Work out the finished part from the listing and answer in its coordinate system (mm). A direction names the side the tool comes from. Coordinates: 2 decimals unless noted, no trailing zeros. Loops run counter-clockwise (first coordinate to the right, second up) from the corner with the lowest first, then second, coordinate; pieces in that order, holes last.
```python
from build123d import *

# Parameters (mm, degrees)
F1_DEPTH       = 7.5
F2_DEPTH       = 2.5
F4_D           = 5.5
F4_DEPTH       = 8
F4_CSINK_D     = 11.2
F4_CSINK_ANGLE = 90
F4_TIP         = 1.6523667023


with BuildPart() as f1:
    # F0 (on Top) → F1 (new body, symmetric)
    with BuildSketch(Plane.XY):
        Polygon((2, 28.0777472107), (2, 40), (-2, 40), (-2, -40), (2, -40), (2, -28.0777472107), (2, -3.9222527893), (2, 3.9222527893), align=None)
    extrude(amount=F1_DEPTH, both=True)

    # F0 (on Top) → F2 (join, symmetric)
    with BuildSketch(Plane.XY):
        with BuildLine():
            Line((21, 28.0777472107), (2, 28.0777472107))
            Line((2, 28.0777472107), (2, 3.9222527893))
            Line((2, 3.9222527893), (21, 3.9222527893))
            Line((21, 3.9222527893), (21, 7.9222527893))
            ThreePointArc((21, 7.9222527893), (6.5, 16), (21, 24.0777472107))
            Line((21, 24.0777472107), (21, 28.0777472107))
        make_face()
        with BuildLine():
            Line((21, -3.9222527893), (2, -3.9222527893))
            Line((2, -3.9222527893), (2, -28.0777472107))
            Line((2, -28.0777472107), (21, -28.0777472107))
            Line((21, -28.0777472107), (21, -24.0777472107))
            ThreePointArc((21, -24.0777472107), (6.5, -16), (21, -7.9222527893))
            Line((21, -7.9222527893), (21, -3.9222527893))
        make_face()
    extrude(amount=F2_DEPTH, both=True)

    # F4
    with Locations(Plane.YZ.offset(2)):
        with Locations((-34.0387472107, 0), (34.0387472107, 0)):
            CounterSinkHole(F4_D / 2, F4_CSINK_D / 2, depth=F4_DEPTH, counter_sink_angle=F4_CSINK_ANGLE)
            with Locations((0, 0, -(F4_DEPTH + F4_TIP / 2))):  # 118° drill point
                Cone(0, F4_D / 2, F4_TIP, mode=Mode.SUBTRACT)


solid = f1.part
```
1. A cutting plane is placed at C-C, the plane y = -16. Give the vertices of the cut face in (x, z).
2. Straight lines are drawn through the part: probe 1 along Y at (x, z) = (-1.3, 0); probe 2 along Y at (x, z) = (16, -1.15); probe 3 along X at (y, z) = (28.5, -6). For each, find the intervals that lie inside material, in ascending order.
3. For faces 5 (the conical face through (-0.712, -36.794, 0.868)), 6 (the flat face through (5, -16, 2.5)), 7 (the flat face through (12, -3.922, 0)), 8 (the flat face through (5, 16, -2.5)), 9 (the cylindrical face through (6.504, -16.283, 0.035)), determine the directions among +Z, -Z, +X, -X, +Y, -Y from which every point of the face is accessible in a straight line to the end or side of a thin tool.
4. Each of these flat-tipped pins is pushed along its axis until it touches: P1, Ø9.5, axis at x = 9.5, y = 15, coming from the -Z side; P2, Ø6, axis at x = 10, z = 1, coming from the +Y side; P3, Ø1.5, axis at x = 8, z = -0.5, coming from the -Y side. Where does it stop, or does it pass through?
5. Determine the mould class of faces 1 (the flat face through (0, -40, 0)), 2 (the cylindrical face through (6.504, 15.717, -0.035)), 3 (the flat face through (11, 3.922, 0)), 4 (the flat face through (21, 26, 0)) for opening direction Y: released by +Y, released by -Y, zero draft, split by the parting line, or undercut.
6. A cutting plane is placed at D-D, the plane x = 0.25. Give the vertices of the cut face in (y, z), then the cut area to 3 significant figures.
7. A cutting plane is placed at A-A, the plane x = 16. Give the vertices of the cut face in (y, z), then the cut area to 3 significant figures.
8. A cutting plane is placed at B-B, the plane z = 0. Give the vertices of the cut face in (x, y), then the cut area to 3 significant figures.
Answers below:
1. outline: (-2, -7.5) - (2, -7.5) - (2, -2.5) - (6.5, -2.5) - (6.5, 2.5) - (2, 2.5) - (2, 7.5) - (-2, 7.5) - close
2. probe 1: y = -40 to -36.79, -31.29 to 31.29, 36.79 to 40
2. probe 2: y = -28.08 to -25.5, -6.5 to -3.92, 3.92 to 6.5, 25.5 to 28.08
2. probe 3: x = -2 to 2
3. face 5: +X
3. face 6: +Z, +X, +Y, -Y
3. face 7: +Z, -Z, +X
3. face 8: -Z, +X, +Y, -Y
3. face 9: +Z, -Z
4. P1: stops at z = -2.5
4. P2: stops at y = 28.08
4. P3: stops at y = -28.08
5. face 1: released by -Y
5. face 2: undercut
5. face 3: undercut
5. face 4: zero draft
6. outline: (-40, -7.5) - (40, -7.5) - (40, 7.5) - (-40, 7.5) - close; hole circle Ø7.7 at (-34.04, 0); hole circle Ø7.7 at (34.04, 0)
6. area: 1,110 mm2
7. outline: (-28.08, -2.5) - (-25.5, -2.5) - (-25.5, 2.5) - (-28.08, 2.5) - close; (-6.5, -2.5) - (-3.92, -2.5) - (-3.92, 2.5) - (-6.5, 2.5) - close; (3.92, -2.5) - (6.5, -2.5) - (6.5, 2.5) - (3.92, 2.5) - close; (25.5, -2.5) - (28.08, -2.5) - (28.08, 2.5) - (25.5, 2.5) - close
7. area: 51.6 mm2
8. outline: (-2, -40) - (2, -40) - (2, -39.64) - (-0.85, -36.79) - (-2, -36.79) - close; (-2, -31.29) - (-0.85, -31.29) - (2, -28.44) - (2, -28.08) - (21, -28.08) - (21, -24.08) arc R9.5 cw (long way) to (21, -7.92) - (21, -3.92) - (2, -3.92) - (2, 3.92) - (21, 3.92) - (21, 7.92) arc R9.5 cw (long way) to (21, 24.08) - (21, 28.08) - (2, 28.08) - (2, 28.44) - (-0.85, 31.29) - (-2, 31.29) - close; (-2, 36.79) - (-0.85, 36.79) - (2, 39.64) - (2, 40) - (-2, 40) - close
8. area: 713 mm2
